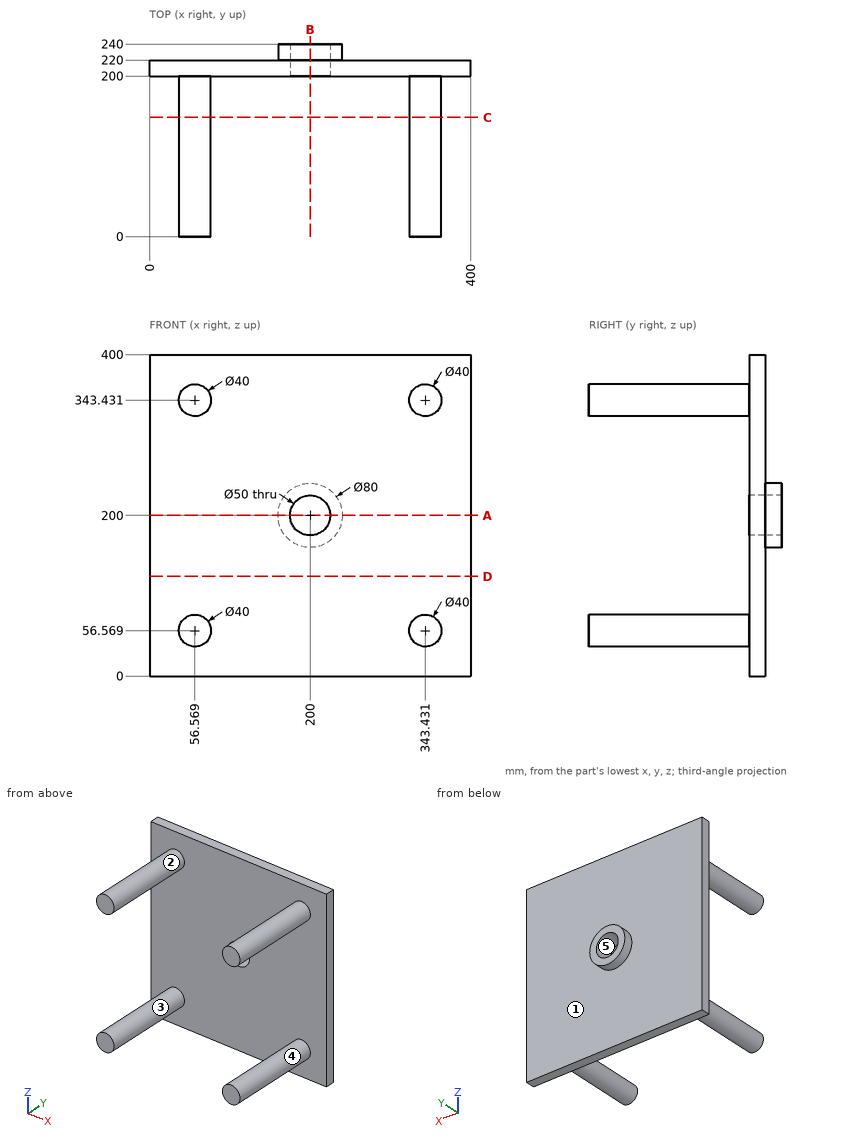
Could you check a few things on this drawing? It's one solid part, dimensions in mm from its lowest x, y, z. A direction names the side the tool comes from. Give positions to 0.01 mm unless a question says otherwise; leave off trailing zeros. Write each loop counter-clockwise with the first axis right and the second up, starting at its lowest first coordinate (ties: lowest second). Pieces come first, ordered by that corner, then holes. Notation, with made-up numbers: (20, -3.5) -> (71, -3.5) arc R30 cw to (71, 32.5) -> close; hole circle Ø7 at (2, -8.5). An arc over 180 degrees is marked (long way). Answer as CSV lines item,"result". Start each with the question number.
(1) I'm going to push flat-ended pins straight in: pin 1 Ø6 at (x, z) = (217.5, 349.5) entering from -Y; pin 2 Ø12 at (x, z) = (40.5, 95.5) entering from +Y. Where does each tip first touch, or does it pass through?
(2) If we section it at C-C, the plane y = 148.5: Write out the boundary of the cut face in (x, z), and give its area (3 significant figures).
(3) Which directions (+Z, -Z, +X, -X, +Y, -Y) give clear straight access to the entire face, cutting with the end or side of a thin tool? Please do the marked faces 4 and 5.
(4) If we section it at D-D, the plane z = 124: Write out the boundary of the cut face in (x, y), and give its area (3 significant figures).
(5) If we section it at A-A, the plane z = 200: Write out the boundary of the cut face in (x, y).
(6) If we section it at B-B, the plane x = 200: Write out the boundary of the cut face in (y, z), and give its area (3 significant figures).
(7) Please list where these lines run through material, in increasing order: line 1 (Z direction, x = 200, y = 214); line 2 (X direction, y = 221, z = 200).
(8) If we mould it in two halves opening along Z, with no side actions, what happens to the marked faces 1, 2 and 3? For each: +Z half, -Z half, draft (parallel to the pull), parting line (faces both ways), or undercut.
Answer list:
1,pin 1,"y = 200"
1,pin 2,"y = 220"
2,outline,"circle Ø40 at (56.57, 56.57); circle Ø40 at (56.57, 343.43); circle Ø40 at (343.43, 56.57); circle Ø40 at (343.43, 343.43)"
2,area,"5,030 mm^2"
3,face 4,"-Y"
3,face 5,"+Y, -Y"
4,outline,"(0, 200) -> (400, 200) -> (400, 220) -> (0, 220) -> close"
4,area,"8,000 mm^2"
5,outline,"(0, 200) -> (175, 200) -> (175, 240) -> (160, 240) -> (160, 220) -> (0, 220) -> close; (225, 200) -> (400, 200) -> (400, 220) -> (240, 220) -> (240, 240) -> (225, 240) -> close"
6,outline,"(200, 0) -> (220, 0) -> (220, 160) -> (240, 160) -> (240, 175) -> (200, 175) -> close; (200, 225) -> (240, 225) -> (240, 240) -> (220, 240) -> (220, 400) -> (200, 400) -> close"
6,area,"7,600 mm^2"
7,line 1,"0 to 175, 225 to 400"
7,line 2,"160 to 175, 225 to 240"
8,face 1,"draft"
8,face 2,"undercut"
8,face 3,"undercut"
